Source: CAD feature listing. Evaluate the final solid. Frame: model axes, mm. Face numbers are marked on the shaded views. Round coordinates to 2 decimals unless told otherwise and drop trailing zeros. Write each loop counter-clockwise with the first axis right and the second up, starting at its lowest first coordinate (ties: lowest second). Pieces come first, ordered by that corner, then holes.
from build123d import *

# Parameters (mm, degrees)
F0_W     = 152.437769
F0_H     = 152.437777
F1_DEPTH = 101.6
F2_R     = 51.98485
F3_DEPTH = 76.2
F4_R     = 34.676264
F5_DEPTH = 177.801


with BuildPart() as f1:
    # F0 (on Top) → F1 (new body)
    with BuildSketch(Plane.XY):
        with Locations((0.220928, -8e-06)):
            Rectangle(F0_W, F0_H)
    extrude(amount=F1_DEPTH)

    # F2 (on face) → F3 (join)
    with BuildSketch(Plane.XY.offset(101.6)):
        Circle(F2_R)
    extrude(amount=F3_DEPTH)

    # F4 (on face) → F5 (cut, through all)
    with BuildSketch(Plane.XY.offset(177.8)):
        Circle(F4_R)
    extrude(amount=-F5_DEPTH, mode=Mode.SUBTRACT)


solid = f1.part
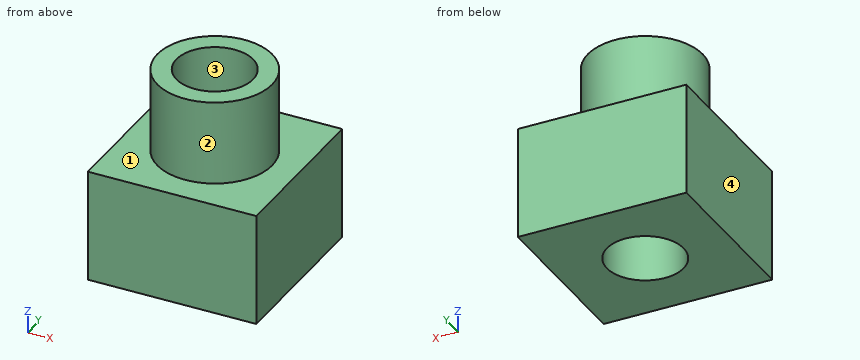
1) Section query D-D on y = 38.5. Return the cut outline in (x, z).
Taken from the geometry:
outline: (-76, 0) - (76.44, 0) - (76.44, 101.6) - (34.93, 101.6) - (34.93, 177.8) - (-34.93, 177.8) - (-34.93, 101.6) - (-76, 101.6) - close
2) Pull-direction query (X, two-part tool) for the marked faces 1, 2, 3 and 4; classes: released by +X, released by -X, zero draft, split by the parting line, or undercut.
Taken from the geometry:
face 1: zero draft
face 2: split by the parting line
face 3: undercut
face 4: released by -X
3) Section query B-B on y = 0. Return the cut outline in (x, z), then the cut area to 3 significant figures.
Taken from the geometry:
outline: (-76, 0) - (-34.68, 0) - (-34.68, 177.8) - (-51.98, 177.8) - (-51.98, 101.6) - (-76, 101.6) - close; (34.68, 0) - (76.44, 0) - (76.44, 101.6) - (51.98, 101.6) - (51.98, 177.8) - (34.68, 177.8) - close
area: 11,100 mm2
4) Section query A-A on x = 0. Return the cut outline in (y, z).
Taken from the geometry:
outline: (-76.22, 0) - (-34.68, 0) - (-34.68, 177.8) - (-51.98, 177.8) - (-51.98, 101.6) - (-76.22, 101.6) - close; (34.68, 0) - (76.22, 0) - (76.22, 101.6) - (51.98, 101.6) - (51.98, 177.8) - (34.68, 177.8) - close
5) Contact query for flat-ended pins moving along their axis: P1, Ø2, axis at y = 39.5, z = 141.5, coming from the +X side; P2, Ø1, axis at x = 19.5, y = -56, coming from the +Z side; P3, Ø1, axis at y = -15, z = 103.5, coming from the -X side. Output: stop coordinate, or through.
Taken from the geometry:
P1: stops at x = 34.93
P2: stops at z = 101.6
P3: stops at x = -49.92
6) Section query C-C on z = 52.5. Return the cut outline in (x, y), then the cut area to 3 significant figures.
Taken from the geometry:
outline: (-76, -76.22) - (76.44, -76.22) - (76.44, 76.22) - (-76, 76.22) - close; hole circle Ø69.35 at (0, 0)
area: 19,500 mm2
7) Material intervals for line 1 (Y direction, x = 0, z = 47.5); line 2 (Z direction, x = 18, y = 65.5); line 3 (Y direction, x = 0, z = 116.5), sorted ascending.
Taken from the geometry:
line 1: y = -76.22 to -34.68, 34.68 to 76.22
line 2: z = 0 to 101.6
line 3: y = -51.98 to -34.68, 34.68 to 51.98
